```python
from build123d import *

# Parameters (mm, degrees)
SKETCH_1_W                   = 41
SKETCH_1_H                   = 15
EXTRUDE_1_DEPTH              = 10
HOLE_WIZARD_M3_1_D           = 3.6
HOLE_WIZARD_M3_1_CBORE_D     = 6.5
HOLE_WIZARD_M3_1_CBORE_DEPTH = 3
SKETCH_4_W                   = 8.5
SKETCH_4_H                   = 6
CUT_EXTRUDE_1_DEPTH          = 45.788391353
SKETCH_5_R                   = 2
CUT_EXTRUDE_2_DEPTH          = 10


with BuildPart() as part:
    # 草图1 → 凸台-拉伸1 (new body)
    with BuildSketch(Plane.XY):
        with Locations((20.5, 7.5)):
            Rectangle(SKETCH_1_W, SKETCH_1_H)
    extrude(amount=EXTRUDE_1_DEPTH)

    # M3 六角凹头螺钉的柱形沉头孔1 (through all)
    with Locations(Plane.XY.offset(10)):
        with Locations((3.5, 7.5), (37.5, 7.5)):
            CounterBoreHole(HOLE_WIZARD_M3_1_D / 2, HOLE_WIZARD_M3_1_CBORE_D / 2, HOLE_WIZARD_M3_1_CBORE_DEPTH)

    # 草图4 → 切除-拉伸1 (cut, through all)
    with BuildSketch(Plane(origin=(0, 15, 0), x_dir=(1, 0, 0), z_dir=(0, 1, 0))):
        with Locations((24.25, -3)):
            Rectangle(SKETCH_4_W, SKETCH_4_H)
    extrude(amount=-CUT_EXTRUDE_1_DEPTH, mode=Mode.SUBTRACT)

    # 草图5 → 切除-拉伸2 (cut)
    with BuildSketch(Plane(origin=(0, 0, 6), x_dir=(-1, 0, 0), z_dir=(0, 0, -1))):
        with Locations((-24.25, 10.8)):
            Circle(SKETCH_5_R)
    extrude(amount=-CUT_EXTRUDE_2_DEPTH, mode=Mode.SUBTRACT)


solid = part.part
```
Can you work these out from the model? Positions are in its coordinate system, mm. A direction names the side the tool comes from. Round coordinates to 2 decimals unless told otherwise and drop trailing zeros. Order: outer loops, then holes, each group sorted by start corner. A loop starts at its lowest first (then second) coordinate and runs counter-clockwise, first axis right, second up. Notation, with made-up numbers: (19.5, 59.5) -> (51.5, 59.5) arc R17 cw to (51.5, 73.5) -> close; hole circle Ø1 at (-10, -3). An arc over 180 degrees is marked (long way). Return JSON: item names as keys, results as strings. Group by question number.
1. If we section it at D-D, the plane y = 10.25: Write out the boundary of the cut face in (x, z).
2. Will these pins go through, and if not, where does the flat tip stop? pin 1 (2.5 mm diameter, centred on x = 26, y = 8, fed in from -Z); pin 2 (6 mm diameter, centred on x = 37.5, y = 7.5, fed in from +Z); pin 3 (2 mm diameter, centred on x = 3.5, y = 7.5, fed in from -Z).
3. Which directions (+Z, -Z, +X, -X, +Y, -Y) give clear straight access to the entire face, cutting with the end or side of a thin tool? Please do faces 1 (the face through (28.5, 8, 3)), 2 (the face through (39, 6, 7)), 3 (the face through (20, 8, 10)).
4. If we section it at A-A, the plane z = 1.25: Write out the boundary of the cut face in (x, y), then the cut area to 3 significant figures.
5. I need wall thicknesses on line 1 (Y direction, x = 3.5, z = 3); line 2 (Y direction, x = 3.5, z = 7.65); line 3 (X direction, y = 11.75, z = 3.25). Which ranges of each line are inside material? Lowest first, please. Write a range as [from, to].
6. We'd pull the mould along X, two halves only. Please class faces 4 (the face through (0, 7, 5)), 5 (the face through (20, 15, 7)), 6 (the face through (3.89, 5.743, 3.451)), 7 (the face through (41, 7, 5)): released by +X, released by -X, zero draft, split by the parting line, or undercut.
7. If we section it at B-B, the plane x = 24.25: Write out the boundary of the cut face in (y, z), then the cut area to 3 significant figures.
8. If we section it at C-C, the plane y = 14: Write out the boundary of the cut face in (x, z), then the cut area to 3 significant figures.
Output values:
{
 "1": {"outline": "(0, 0) -> (20, 0) -> (20, 6) -> (22.33, 6) -> (22.33, 10) -> (5.23, 10) -> (5.23, 7) -> (1.77, 7) -> (1.77, 10) -> (0, 10) -> close; (26.17, 6) -> (28.5, 6) -> (28.5, 0) -> (41, 0) -> (41, 10) -> (39.23, 10) -> (39.23, 7) -> (35.77, 7) -> (35.77, 10) -> (26.17, 10) -> close"},
 "2": {"pin 1": "z = 6", "pin 2": "z = 7", "pin 3": "through"},
 "3": {"face 1": "-Z, +Y, -Y", "face 2": "+Z", "face 3": "+Z, +X, -X, +Y, -Y"},
 "4": {"outline": "(0, 0) -> (20, 0) -> (20, 15) -> (0, 15) -> close; (28.5, 0) -> (41, 0) -> (41, 15) -> (28.5, 15) -> close; hole circle Ø3.6 at (3.5, 7.5); hole circle Ø3.6 at (37.5, 7.5)", "area": "467 mm²"},
 "5": {"line 1": "[0, 5.7], [9.3, 15]", "line 2": "[0, 4.25], [10.75, 15]", "line 3": "[0, 20], [28.5, 41]"},
 "6": {"face 4": "released by -X", "face 5": "zero draft", "face 6": "undercut", "face 7": "released by +X"},
 "7": {"outline": "(0, 6) -> (8.8, 6) -> (8.8, 10) -> (0, 10) -> close; (12.8, 6) -> (15, 6) -> (15, 10) -> (12.8, 10) -> close", "area": "44.0 mm²"},
 "8": {"outline": "(0, 0) -> (20, 0) -> (20, 6) -> (28.5, 6) -> (28.5, 0) -> (41, 0) -> (41, 10) -> (0, 10) -> close", "area": "359 mm²"}
}
